Autodesk Inventor part; units mm, degrees
ref_plane "YZ Plane" through (0, 0, 0) normal (1, 0, 0) x (0, 1, 0)
ref_plane "XZ Plane" through (0, 0, 0) normal (0, 1, 0) x (-1, 0, 0)
ref_plane "XY Plane" through (0, 0, 0) normal (0, 0, 1) x (1, 0, 0)
sketch "Sketch1" plane through (0, 0, 0) normal (0, 1, 0) x (-1, 0, 0)
  circle A0 centre (0, 0) radius 7.5
  dimension "d0" = 15
extrude "Extrusion1" add sketch "Sketch1" along normal blind 6
sketch "Sketch2" plane through (0, 0, 0) normal (0, -1, 0) x (1, 0, 0)
  circle A0 centre (0, 0) radius 7.5
hole "Hole1" at (0, 0, 0) direction (0, 1, 0) diameter 4.917 end through all
chamfer "Chamfer1" distance 0.5 angle 45 1 edges at (0, 0, 2.4585)
properties part number "02-13-docisk_K3" material "Stainless Steel"
Verification items for the finished model (mm, model axes). Give positions to 0.01 mm unless a question says otherwise; leave off trailing zeros. Loops run counter-clockwise (first coordinate to the right, second up) from the corner with the lowest first, then second, coordinate; pieces in that order, holes last.
1) Depth check by flat-ended pin: pin 1 Ø1.5 at (y, z) = (5, -3.5) entering from +X; pin 2 Ø1 at (y, z) = (1.5, 4) entering from -X; pin 3 Ø1 at (x, y) = (1, 4) entering from +Z. Enter the tip coordinate at first touch or a pass-through.
2) Sectioned sample at B-B, the plane z = 0. Enter the section's corners in (x, y).
3) Draft check along Z on faces 1 (the cylindrical face through (-0.738, 3.288, -2.345)), 2 (the cylindrical face through (7.493, 2.958, -0.33)), 3 (the flat face through (2, 6, 2)). Enter one of: pulls with the +Z half, pulls with the -Z half, needs draft (parallel to the pull), parting line crosses it, or undercut.
4) Sectioned sample at D-D, the plane z = -4.5. Enter the section's corners in (x, y), then the cut area to 3 significant figures.
5) Thickness scan on line 1 along Z through (x, y) = (0, 2.85); line 2 along Z through (x, y) = (-1.75, 4.1). Record the ranges inside material, lowest first.
6) Sectioned sample at A-A, the plane x = 0. Enter the section's corners in (y, z), then the cut area to 3 significant figures.
7) Sectioned sample at C-C, the plane y = 3.55. Enter the section's corners in (x, z), then the cut area to 3 significant figures.
Answers:
1. pin 1: stops at x = 6.98
1. pin 2: stops at x = -6.63
1. pin 3: stops at z = 7.48
2. outline: (-7.5, 0) - (-2.96, 0) - (-2.46, 0.5) - (-2.46, 6) - (-7.5, 6) - close; (2.46, 0.5) - (2.96, 0) - (7.5, 0) - (7.5, 6) - (2.46, 6) - close
3. face 1: undercut
3. face 2: parting line crosses it
3. face 3: needs draft
4. outline: (-6, 0) - (6, 0) - (6, 6) - (-6, 6) - close
4. area: 72.0 mm2
5. line 1: z = -7.5 to -2.46, 2.46 to 7.5
5. line 2: z = -7.29 to -1.73, 1.73 to 7.29
6. outline: (0, -7.5) - (6, -7.5) - (6, -2.46) - (0.5, -2.46) - (0, -2.96) - close; (0, 2.96) - (0.5, 2.46) - (6, 2.46) - (6, 7.5) - (0, 7.5) - close
6. area: 60.2 mm2
7. outline: circle Ø15 at (0, 0); hole circle Ø4.92 at (0, 0)
7. area: 158 mm2
